Verification items for the finished model (mm, model axes). Face numbers are marked on the shaded views. A direction names the side the tool comes from. Give positions to 0.01 mm unless a question says otherwise; leave off trailing zeros. Order: outer loops, then holes, each group sorted by start corner. A loop starts at its lowest first (then second) coordinate and runs counter-clockwise, first axis right, second up.
(1) Gauge pin test, flat end, axial feed: pin 1 (12 mm diameter, centred on x = -26, y = 1, fed in from +Z). Record the tip position at first contact, or that the pin passes through.
(2) Access from +Z, -Z, +X, -X, +Y, -Y to the whole of each face (thin tool, end or side, straight path). Record for the marked faces 1 and 2.
(3) Sectioned sample at C-C on y = 18.5. Record the cut outline in (x, z).
(4) Sectioned sample at D-D on x = 18. Record the cut outline in (y, z).
(5) Scan lines: L1, parallel to X at y = -11.5, z = 26; L2, parallel to Y at x = -26, z = 10; L3, parallel to Z at x = -20, y = -20.5. Record each from-to range of solid material in increasing order.
(6) Sectioned sample at B-B on z = 25.5. Record the cut outline in (x, y).
(7) Mould release check, pull along X, two halves, no side actions. Record for the marked faces 3, 4, 5 and 6: pulls with the +X half, pulls with the -X half, needs draft (parallel to the pull), parting line crosses it, or undercut.
(8) Sectioned sample at A-A on y = -11. Record the cut outline in (x, z), plus the area to 3 significant figures.
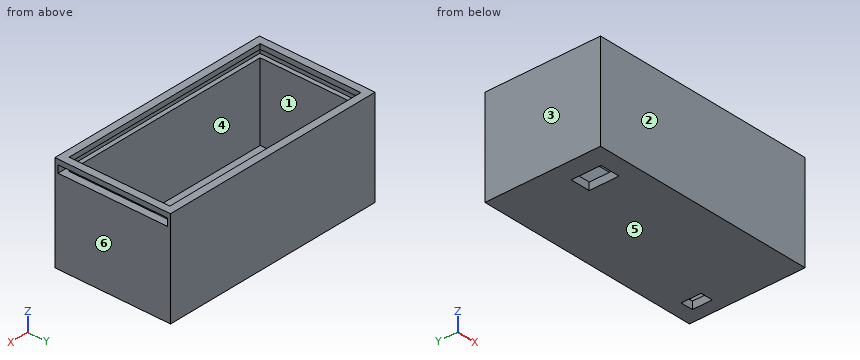
```python
from build123d import *

# Parameters (mm, degrees)
SKETCH_1_W          = 91
SKETCH_1_H          = 46.5
SKETCH_1_W_2        = 85
SKETCH_1_H_2        = 40.5
EXTRUDE_1_DEPTH     = 36
SKETCH_2_W          = 91
SKETCH_2_H          = 46.5
EXTRUDE_2_DEPTH     = 3
SKETCH_3_W          = 90
SKETCH_3_H          = 44
CUT_EXTRUDE_1_DEPTH = 3
SKETCH_4_W          = 8
SKETCH_4_H          = 12
SKETCH_4_W_2        = 5
SKETCH_4_H_2        = 8
CUT_EXTRUDE_2_DEPTH = 10


with BuildPart() as part:
    # 草圖1 → 填料-伸長1 (new body)
    with BuildSketch(Plane.XY):
        Rectangle(SKETCH_1_W, SKETCH_1_H)
        Rectangle(SKETCH_1_W_2, SKETCH_1_H_2, mode=Mode.SUBTRACT)
    extrude(amount=EXTRUDE_1_DEPTH)

    # 草圖2 → 填料-伸長2 (add)
    with BuildSketch(Plane(origin=(0, 0, 0), x_dir=(-1, 0, 0), z_dir=(0, 0, -1))):
        Rectangle(SKETCH_2_W, SKETCH_2_H)
    extrude(amount=EXTRUDE_2_DEPTH)

    # 草圖3 → 除料-伸長1 (cut)
    with BuildSketch(Plane.XY.offset(31)):
        with Locations((0.75, 0)):
            Rectangle(SKETCH_3_W, SKETCH_3_H)
    extrude(amount=CUT_EXTRUDE_1_DEPTH, mode=Mode.SUBTRACT)

    # 草圖4 → 除料-伸長2 (cut)
    with BuildSketch(Plane(origin=(0, 0, -3), x_dir=(-1, 0, 0), z_dir=(0, 0, -1))):
        with Locations((33.5, -10.25)):
            Rectangle(SKETCH_4_W, SKETCH_4_H)
        with Locations((-37.648642632, 13.25)):
            Rectangle(SKETCH_4_W_2, SKETCH_4_H_2)
    extrude(amount=-CUT_EXTRUDE_2_DEPTH, mode=Mode.SUBTRACT)


solid = part.part
```
Ans:
1. pin 1: stops at z = 0
2. face 1: +Z
2. face 2: +Z, -Z, +X, -X, -Y
3. outline: (-45.5, -3) - (45.5, -3) - (45.5, 31) - (42.5, 31) - (42.5, 0) - (-42.5, 0) - (-42.5, 31) - (-44.25, 31) - (-44.25, 34) - (-42.5, 34) - (-42.5, 36) - (-45.5, 36) - close; (42.5, 34) - (45.5, 34) - (45.5, 36) - (42.5, 36) - close
4. outline: (-23.25, -3) - (23.25, -3) - (23.25, 36) - (20.25, 36) - (20.25, 34) - (22, 34) - (22, 31) - (20.25, 31) - (20.25, 0) - (-20.25, 0) - (-20.25, 31) - (-22, 31) - (-22, 34) - (-20.25, 34) - (-20.25, 36) - (-23.25, 36) - close
5. L1: x = -45.5 to -42.5, 42.5 to 45.5
5. L2: y = -23.25 to -20.25, 20.25 to 23.25
5. L3: z = -3 to 31, 34 to 36
6. outline: (-45.5, -23.25) - (45.5, -23.25) - (45.5, 23.25) - (-45.5, 23.25) - close; hole (-42.5, -20.25) - (42.5, -20.25) - (42.5, 20.25) - (-42.5, 20.25) - close
7. face 3: pulls with the -X half
7. face 4: undercut
7. face 5: needs draft
7. face 6: pulls with the +X half
8. outline: (-45.5, -3) - (-37.5, -3) - (-37.5, 0) - (-42.5, 0) - (-42.5, 31) - (-44.25, 31) - (-44.25, 34) - (-42.5, 34) - (-42.5, 36) - (-45.5, 36) - close; (-29.5, -3) - (45.5, -3) - (45.5, 31) - (42.5, 31) - (42.5, 0) - (-29.5, 0) - close; (42.5, 34) - (45.5, 34) - (45.5, 36) - (42.5, 36) - close
8. area: 451 mm2
